from build123d import *

# Parameters (mm, degrees)
BOSS_EXTRUDE1_DEPTH            = 35
SKETCH2_R                      = 1.65
BOSS_EXTRUDE2_DEPTH            = 9
BOSS_EXTRUDE3_DEPTH            = 10.5
SKETCH5_R                      = 19.5
CUT_EXTRUDE1_DEPTH             = 3
FILLET1_R                      = 5
FILLET2_R                      = 2
F_4_0MM_DOWEL_HOLE2_AT_2_COUNT = 2
F_4_0MM_DOWEL_HOLE2_AT_2_PITCH = 30
F_4_0MM_DOWEL_HOLE2_AT_3_COUNT = 2
F_4_0MM_DOWEL_HOLE2_AT_3_PITCH = 30


with BuildPart() as part:
    # Sketch1 → Boss-Extrude1 (new body)
    with BuildSketch(Plane.XY):
        Polygon((-45, 7), (-45, -12), (45, -12), (45, 7), (40, 7), (40, -7), (-40, -7), (-40, 7), align=None)
    extrude(amount=BOSS_EXTRUDE1_DEPTH)

    # Sketch2 → Boss-Extrude2 (add)
    with BuildSketch(Plane.XY.offset(35)):
        with BuildLine():
            Line((-45, 33), (-45, -12))
            Line((-45, -12), (-20, -12))
            Line((-20, -12), (-21.669336841, 3.024031571))
            ThreePointArc((-21.669336841, 3.024031571), (-26.926604816, 11.674821687), (-23.696516817, 21.268651356))
            Line((-23.696516817, 21.268651356), (-25, 33))
            Line((-25, 33), (-45, 33))
        make_face()
        with Locations((-30.5, 8)):
            Circle(SKETCH2_R, mode=Mode.SUBTRACT)
        with Locations((-30.5, 18)):
            Circle(SKETCH2_R, mode=Mode.SUBTRACT)
    boss_extrude2 = extrude(amount=BOSS_EXTRUDE2_DEPTH)

    # Mirror2: Boss-Extrude2 across plane
    add(boss_extrude2.mirror(Plane(origin=(-5.25, 13.784906966, -116.647939609), x_dir=(0, 0, 1), z_dir=(-1, 0, 0))))

    # Sketch4 → Boss-Extrude3 (add)
    with BuildSketch(Plane(origin=(34.5, 0, 0), x_dir=(0, 0, -1), z_dir=(1, 0, 0))):
        Polygon((-35, -7), (-35, 33), (-44, 33), (-44, -12), (-35, -12), align=None)
    extrude(amount=BOSS_EXTRUDE3_DEPTH)

    # Sketch5 → Cut-Extrude1 (cut)
    with BuildSketch(Plane(origin=(0, 0, 35), x_dir=(-1, 0, 0), z_dir=(0, 0, -1))):
        with Locations((-4.5, 13)):
            Circle(SKETCH5_R)
    extrude(amount=-CUT_EXTRUDE1_DEPTH, mode=Mode.SUBTRACT)

    # Fillet1
    fillet1_edges = [part.edges().sort_by_distance(p)[0] for p in [
        (45, -12, 22),
        (-45, -12, 22),
        (-40, -7, 17.5),
        (40, -7, 17.5),
    ]]
    fillet(fillet1_edges, radius=FILLET1_R)

    # Fillet2
    fillet2_edges = [part.edges().sort_by_distance(p)[0] for p in [
        (-5.25, -12, 35),
        (-45, 33, 39.5),
        (-25, 33, 39.5),
        (45, 33, 39.5),
        (-42.5, 7, 0),
        (42.5, 7, 0),
        (14.5, 33, 39.5),
        (9.777777778, -9.5, 35),
        (-20.277777778, -9.5, 35),
        (-20, -12, 39.5),
        (9.5, -12, 39.5),
    ]]
    fillet(fillet2_edges, radius=FILLET2_R)

    # Sketch6 → Ø4.0mm Dowel Hole2 (revolve, cut)
    with BuildSketch(Plane(origin=(0, -12, 4), x_dir=(0, 0, -1), z_dir=(1, 0, 0))):
        Polygon((0, 0), (0, 5), (2.025, 5), (2, 4.975), (2, 0.025), (2.025, 0), align=None)
    f_4_0mm_dowel_hole2 = revolve(axis=Axis((0, -18.35, 4), (0, 1, 0)), mode=Mode.SUBTRACT)

    # Ø4.0mm Dowel Hole2 at 2: Ø4.0mm Dowel Hole2 ×2
    with Locations(*[(i * F_4_0MM_DOWEL_HOLE2_AT_2_PITCH, 0, 0) for i in range(1, F_4_0MM_DOWEL_HOLE2_AT_2_COUNT)]):
        add(f_4_0mm_dowel_hole2, mode=Mode.SUBTRACT)

    # Ø4.0mm Dowel Hole2 at 3: Ø4.0mm Dowel Hole2 ×2
    with Locations(*[(-i * F_4_0MM_DOWEL_HOLE2_AT_3_PITCH, 0, 0) for i in range(1, F_4_0MM_DOWEL_HOLE2_AT_3_COUNT)]):
        add(f_4_0mm_dowel_hole2, mode=Mode.SUBTRACT)

    # Sketch9 → Ø4.0mm Dowel Hole3 (revolve, cut)
    with BuildSketch(Plane(origin=(45, 1, 4), x_dir=(0, 0, -1), z_dir=(0, 1, 0))):
        Polygon((0, 0), (0, 5), (2.025, 5), (2, 4.975), (2, 0.025), (2.025, 0), align=None)
    f_4_0mm_dowel_hole3 = revolve(axis=Axis((51.35, 1, 4), (-1, 0, 0)), mode=Mode.SUBTRACT)

    # Mirror3: Ø4.0mm Dowel Hole3 across plane
    add(f_4_0mm_dowel_hole3.mirror(Plane(origin=(0, 0, 0), x_dir=(0, 0, 1), z_dir=(1, 0, 0))), mode=Mode.SUBTRACT)

    # Mirror4: Ø4.0mm Dowel Hole2, Ø4.0mm Dowel Hole3 across plane
    add(f_4_0mm_dowel_hole2.mirror(Plane(origin=(0, 0, 17.5), x_dir=(1, 0, 0), z_dir=(0, 0, -1))), mode=Mode.SUBTRACT)
    add(f_4_0mm_dowel_hole3.mirror(Plane(origin=(0, 0, 17.5), x_dir=(1, 0, 0), z_dir=(0, 0, -1))), mode=Mode.SUBTRACT)

    # Mirror4 copy 1 sketch → Mirror4 copy 1 (revolve, cut)
    with BuildSketch(Plane(origin=(30, -12, 31), x_dir=(0, 0, 1), z_dir=(1, 0, 0))):
        Polygon((0, 0), (0, -5), (2.025, -5), (2, -4.975), (2, -0.025), (2.025, 0), align=None)
    revolve(axis=Axis((30, -18.35, 31), (0, -1, 0)), mode=Mode.SUBTRACT)

    # Mirror4 copy 2 sketch → Mirror4 copy 2 (revolve, cut)
    with BuildSketch(Plane(origin=(-30, -12, 31), x_dir=(0, 0, 1), z_dir=(1, 0, 0))):
        Polygon((0, 0), (0, -5), (2.025, -5), (2, -4.975), (2, -0.025), (2.025, 0), align=None)
    revolve(axis=Axis((-30, -18.35, 31), (0, -1, 0)), mode=Mode.SUBTRACT)

    # Mirror4 copy 3 sketch → Mirror4 copy 3 (revolve, cut)
    with BuildSketch(Plane(origin=(-45, 1, 31), x_dir=(0, 0, 1), z_dir=(0, 1, 0))):
        Polygon((0, 0), (0, 5), (2.025, 5), (2, 4.975), (2, 0.025), (2.025, 0), align=None)
    revolve(axis=Axis((-51.35, 1, 31), (1, 0, 0)), mode=Mode.SUBTRACT)


solid = part.part
Work out the finished part from the listing and answer in its coordinate system (mm). A direction names the side the tool comes from. Round coordinates to 2 decimals unless told otherwise and drop trailing zeros. Write each loop counter-clockwise with the first axis right and the second up, starting at its lowest first coordinate (ties: lowest second). Pieces come first, ordered by that corner, then holes. Notation, with made-up numbers: (42.5, 16) - (92.5, 16) arc R22 cw to (92.5, 27) - close; hole circle Ø7 at (-28.5, 84). An arc over 180 degrees is marked (long way). Answer in a Markdown table with one row per item. Add a question column.
1. A cutting plane is placed at A-A, the plane z = 39.5. Determine the outline of the cut face in (x, y), and give its area (3 significant figures).
2. A cutting plane is placed at D-D, the plane x = -30. Count the separate pieces of the cut face and the enclosed holes in it, and give its area (3 significant figures).
3. A cutting plane is placed at C-C, the plane y = 11. Determine the outline of the cut face in (x, z).
4. For faces 1 (the flat face through (0, -7, 18)), 2 (the cylindrical face through (-25.441, 32.477, 39.563)), 3 (the cylindrical face through (44.43, 32.4, 39.56)), determine the directions among +Z, -Z, +X, -X, +Y, -Y from which every point of the face is accessible in a straight line to the end or side of a thin tool.
5. Given pin 1 (3.5 mm diameter, centred on x = -30, z = 31, fed in from +Y); pin 2 (5 mm diameter, centred on x = 12, y = -2, fed in from -Z); pin 3 (4 mm diameter, centred on x = -30.5, y = 18, fed in from +Z); pin 4 (4 mm diameter, centred on x = -32.5, z = 11, fed in from +Y), each flat-ended and moving along its own axis, determine where each tip first touches the part or whether it passes through.
6. Find the intervals of material crossed by line 1 along Z through (x, y) = (-30, -9); line 2 along Z through (x, y) = (0, -8); line 3 along X through (y, z) = (-9.55, 4), in increasing order. Write a range as from..to.
7. A cutting plane is placed at B-B, the plane x = 30. Determine the outline of the cut face in (y, z) (3 decimals), and give its area (3 significant figures).
8. The mould has two halves that part along Y. Classify faces 4 (the cylindrical face through (-26.91, 11.53, 39.44)), 5 (the flat face through (10.448, -3.467, 40.437)), 6 (the cylindrical face through (16.41, 11.53, 40.96)), 7 (the flat face through (-45, 4, 27)): +Y half, -Y half, draft (parallel to the pull), parting line (faces both ways), or undercut.
Worked out:
| question | item | result |
|---|---|---|
| 1 | outline | (-45, -7) arc R5 ccw to (-40, -12) - (-22.23, -12) arc R2 ccw to (-20.25, -9.78) - (-21.67, 3.02) arc R12 cw to (-23.7, 21.27) - (-24.8, 31.22) arc R2 ccw to (-26.79, 33) - (-43, 33) arc R2 ccw to (-45, 31) - close; (9.75, -9.78) arc R2 ccw to (11.73, -12) - (40, -12) arc R5 ccw to (45, -7) - (45, 31) arc R2 ccw to (43, 33) - (16.29, 33) arc R2 ccw to (14.3, 31.22) - (13.2, 21.27) arc R12 cw to (11.17, 3.02) - close; hole circle Ø3.3 at (-30.5, 8); hole circle Ø3.3 at (-30.5, 18); hole circle Ø3.3 at (20, 8); hole circle Ø3.3 at (20, 18) |
| 1 | area | 2,340 mm^2 |
| 2 | separate pieces | 5 |
| 2 | enclosed holes | 0 |
| 2 | area | 483 mm^2 |
| 3 | outline | (-45, 35) - (-26.83, 35) - (-26.83, 44) - (-45, 44) - close; (16.33, 38) - (23.9, 38) - (23.9, 35) - (45, 35) - (45, 44) - (16.33, 44) - close |
| 4 | face 1 | -Z, +Y |
| 4 | face 2 | +Z, -Z, +Y |
| 4 | face 3 | +Z, -Z, +X, +Y |
| 5 | pin 1 | through |
| 5 | pin 2 | z = 38 |
| 5 | pin 3 | z = 44 |
| 5 | pin 4 | y = -7 |
| 6 | line 1 | 0..2, 6..29, 33..44 |
| 6 | line 2 | 0..2, 6..29, 33..35 |
| 6 | line 3 | -44.3..-32, -28..-2, 2..28, 32..44.3 |
| 7 | outline | (-12, 0) - (-7, 0) - (-7, 1.975) - (-7.025, 2) - (-11.975, 2) - (-12, 1.975) - close; (-12, 6.025) - (-11.975, 6) - (-7.025, 6) - (-7, 6.025) - (-7, 28.975) - (-7.025, 29) - (-11.975, 29) - (-12, 28.975) - close; (-12, 33.025) - (-11.975, 33) - (-7.025, 33) - (-7, 33.025) - (-7, 35) - (33, 35) - (33, 44) - (-12, 44) - close |
| 7 | area | 540 mm^2 |
| 8 | face 4 | undercut |
| 8 | face 5 | +Y half |
| 8 | face 6 | undercut |
| 8 | face 7 | draft |
